```python
from build123d import *

# Parameters (mm, degrees)
SKETCH001_W  = 0.5
SKETCH001_H  = 6.25
PAD_DEPTH    = 20
SKETCH002_W  = 6
SKETCH002_H  = 10.057596
PAD001_DEPTH = 5


with BuildPart() as part:
    # Sketch → Revolution (revolve)
    with BuildSketch(Plane.XZ):
        Polygon((0, 0), (7.25, 0), (4.452154, 6), (4.452154, 15), (7.25, 21), (0, 21), align=None)
    revolve(axis=Axis((0, 0, 0), (0, 0, 1)))

    # Sketch001 → Pad (new body)
    with BuildSketch(Plane(origin=(0, 0, 21), x_dir=(-1, 0, 0), z_dir=(0, 0, 1))):
        with Locations((-2.5, 1)):
            Rectangle(SKETCH001_W, SKETCH001_H)
    extrude(amount=-PAD_DEPTH)

    # Sketch002 → Pad001 (new body)
    with BuildSketch(Plane.XZ.offset(4.125)):
        with Locations((5.25, 10.5)):
            Rectangle(SKETCH002_W, SKETCH002_H)
    extrude(amount=-PAD001_DEPTH)


solid = part.part
```
Geometry check sheet. Reference: the model listing, model coordinates, mm. A direction names the side the tool comes from. Give positions to 0.01 mm unless a question says otherwise; leave off trailing zeros. Order: outer loops, then holes, each group sorted by start corner. A loop starts at its lowest first (then second) coordinate and runs counter-clockwise, first axis right, second up. Notation, with made-up numbers: (8, 27.5) -> (50, 27.5) arc R22 ccw to (50, 64.5) -> close; hole circle Ø11 at (17.25, 7.5). An arc over 180 degrees is marked (long way). Write each question's results on one line, items separated by ' | '. Start each with the question number.
(1) Sectioned sample at A-A (x = 0). Enter the section's corners in (y, z).
(2) Scan lines: line 1 (Z direction, x = 6.5, y = -1.5); line 2 (Z direction, x = 0.75, y = -5.25); line 3 (Z direction, x = 2.25, y = 4). Record each from-to range of solid material in increasing order.
(3) Gauge pin test, flat ends, axial feed: P1, Ø3, axis at x = 4, z = 9, coming from the +Y side; P2, Ø6.5, axis at x = 4.5, z = 11, coming from the -Y side; P3, Ø2, axis at x = 2.5, z = 2.5, coming from the +Y side. Record the tip position at first contact, or that the pin passes through.
(4) Sectioned sample at B-B (z = 8). Enter the section's corners in (x, y) (3 decimals).
(5) Mould release check, pull along Z, two halves, no side actions. Record for faces 1 (the face through (6, -2, 5.471)), 2 (the face through (0, 0, 0)), 3 (the face through (0, 0, 21)): pulls with the +Z half, pulls with the -Z half, needs draft (parallel to the pull), parting line crosses it, or undercut.
(6) Sectioned sample at C-C (y = 0). Enter the section's corners in (x, z), plus the area to 3 significant figures.
(7) Access from +Z, -Z, +X, -X, +Y, -Y to the whole of each face (thin tool, end or side, straight path). Record for faces 4 (the face through (5, -4.125, 11)), 5 (the face through (-3.64, 3.337, 16.042)), 6 (the face through (6, 0.875, 11)).
(8) Sectioned sample at D-D (z = 18.5). Enter the section's corners in (x, y).
Answer below:
1) outline: (-7.25, 0) -> (7.25, 0) -> (4.45, 6) -> (4.45, 15) -> (7.25, 21) -> (-7.25, 21) -> (-4.45, 15) -> (-4.45, 6) -> close
2) line 1: 0 to 1.24, 5.47 to 15.53, 19.76 to 21 | line 2: 0 to 4.17, 16.83 to 21 | line 3: 0 to 5.71, 15.29 to 21
3) P1: y = 3.68 | P2: y = -4.27 | P3: y = 6.17
4) outline: (2.25, -4.125) -> (8.25, -4.125) -> (8.25, 0.875) -> (4.365, 0.875) arc R4.452 ccw (long way) to (2.25, -3.842) -> close
5) face 1: undercut | face 2: pulls with the -Z half | face 3: pulls with the +Z half
6) outline: (-7.25, 0) -> (7.25, 0) -> (4.7, 5.47) -> (8.25, 5.47) -> (8.25, 15.53) -> (4.7, 15.53) -> (7.25, 21) -> (-7.25, 21) -> (-4.45, 15) -> (-4.45, 6) -> close | area: 259 mm2
7) face 4: +X, -Y | face 5: none | face 6: +X, +Y
8) outline: circle Ø12.17 at (0, 0)
